Print and shaded views of the part. All mm, measured from the part's lowest x, y and z. A direction names the side the tool comes from. Round coordinates to 2 decimals unless told otherwise and drop trailing zeros. Write each loop counter-clockwise with the first axis right and the second up, starting at its lowest first coordinate (ties: lowest second). Pieces come first, ordered by that corner, then holes.
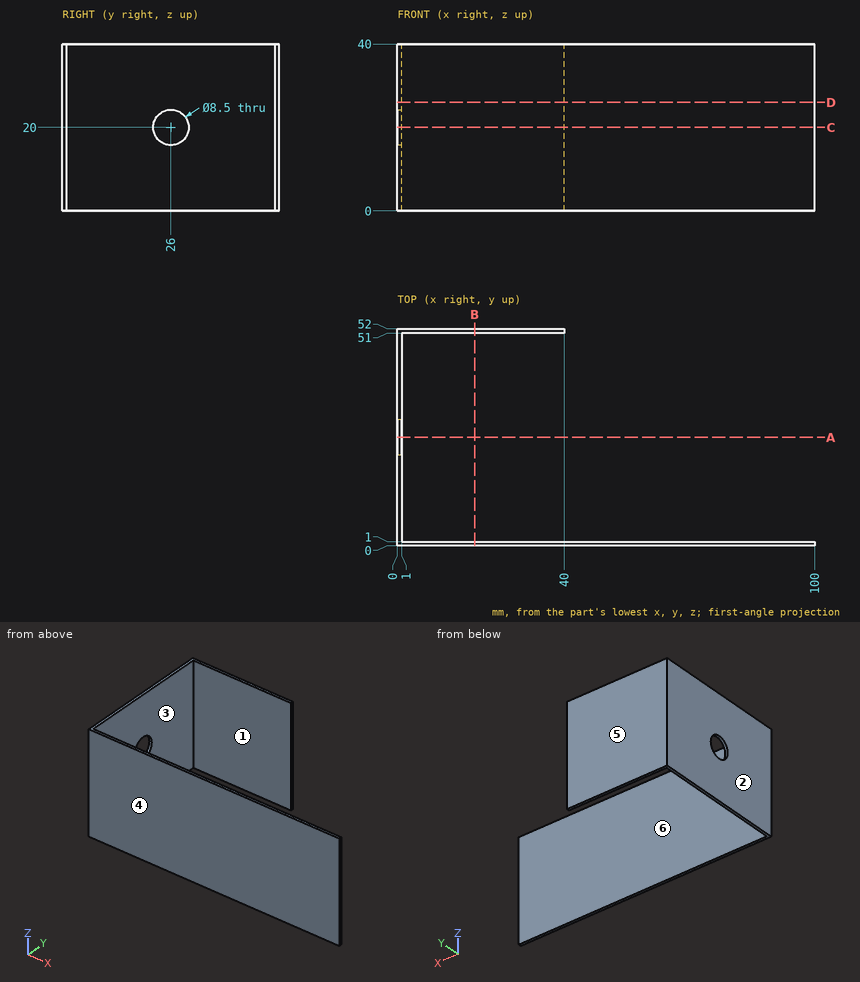
1) Slice it at D-D (z = 26). Write the cut outline in (x, y).
Results:
outline: (0, 0) - (100, 0) - (100, 1) - (1, 1) - (1, 51) - (40, 51) - (40, 52) - (0, 52) - close
2) Wall check: L1, parallel to Y at x = 12.5, z = 31; L2, parallel to Y at x = 0.45, z = 20; L3, parallel to X at y = 49, z = 5.5. Give the ranges that are in metal, low to high.
Results:
L1: y = 0 to 1, 51 to 52
L2: y = 0 to 21.75, 30.25 to 52
L3: x = 0 to 1
3) Mould opens along Y. For the marked faces 3, 4, 5 and 6 say: released by +Y, released by -Y, zero draft, split by the parting line, or undercut.
Results:
face 3: undercut
face 4: released by -Y
face 5: released by +Y
face 6: undercut
4) Which spindle directions (+Z, -Z, +X, -X, +Y, -Y) get a long thin tool onto all of the face, cutting with end or side? Do the marked faces 1 and 2. Say none if no direction does.
Results:
face 1: +Z, -Z, +X
face 2: +Z, -Z, -X, +Y, -Y
5) Slice it at C-C (z = 20). Write the cut outline in (x, y).
Results:
outline: (0, 0) - (100, 0) - (100, 1) - (1, 1) - (1, 21.75) - (0, 21.75) - close; (0, 30.25) - (1, 30.25) - (1, 51) - (40, 51) - (40, 52) - (0, 52) - close
6) Pin check, flat tips, straight feed: pin 1 Ø12 at (y, z) = (26, 29.5) entering from +X; pin 2 Ø20 at (x, z) = (69.5, 23.5) entering from +Y; pin 3 Ø0.5 at (y, z) = (51.5, 29) entering from +X. Stop position of each tip, or through.
Results:
pin 1: stops at x = 1
pin 2: stops at y = 1
pin 3: stops at x = 40
7) Slice it at A-A (y = 26). Write the cut outline in (x, z), plus the area to 3 significant figures.
Results:
outline: (0, 0) - (1, 0) - (1, 15.75) - (0, 15.75) - close; (0, 24.25) - (1, 24.25) - (1, 40) - (0, 40) - close
area: 31.5 mm2
8) Slice it at B-B (x = 18.5). Write the cut outline in (y, z).
Results:
outline: (0, 0) - (1, 0) - (1, 40) - (0, 40) - close; (51, 0) - (52, 0) - (52, 40) - (51, 40) - close
